```python
from build123d import *

# Parameters (mm, degrees)
SKETCH1_R                = 0.75
BOSS_EXTRUDE1_DEPTH      = 10
BOSS_EXTRUDE2_DEPTH      = 1.5
BOSS_EXTRUDE2_DEPTH_BACK = 1.5
FILLET1_R                = 1
SKETCH3_R                = 0.6
CUT_EXTRUDE1_DEPTH       = 5


with BuildPart() as part:
    # Sketch1 → Boss-Extrude1 (new body)
    with BuildSketch(Plane(origin=(0, 0, 0), x_dir=(0, 0, -1), z_dir=(1, 0, 0))):
        Circle(SKETCH1_R)
    extrude(amount=BOSS_EXTRUDE1_DEPTH)

    # Sketch2 → Boss-Extrude2 (add, two sides: drawn at the far end of the back side and taken through both)
    with BuildSketch(Plane(origin=(0, 0, 0), x_dir=(1, 0, 0), z_dir=(0, 1, 0)).offset(-BOSS_EXTRUDE2_DEPTH_BACK)):
        Polygon((1, 1.875), (1, -1.875), (-3, -1.875), (-3, -0.875), (0, -0.875), (0, 0.875), (-3, 0.875), (-3, 1.875), align=None)
    extrude(amount=BOSS_EXTRUDE2_DEPTH + BOSS_EXTRUDE2_DEPTH_BACK)

    # Fillet1
    fillet1_edges = [part.edges().sort_by_distance(p)[0] for p in [
        (-3, 1.5, 1.375),
        (-3, 1.5, -1.375),
        (-3, -1.5, -1.375),
        (1, 0, -1.875),
        (1, 0, 1.875),
        (-3, -1.5, 1.375),
    ]]
    fillet(fillet1_edges, radius=FILLET1_R)

    # Sketch3 → Cut-Extrude1 (cut)
    with BuildSketch(Plane(origin=(0, 0, -1.875), x_dir=(-1, 0, 0), z_dir=(0, 0, -1))):
        with Locations((1.7, 0)):
            Circle(SKETCH3_R)
    extrude(amount=-CUT_EXTRUDE1_DEPTH, mode=Mode.SUBTRACT)


solid = part.part
```
Work out the finished part from the listing and answer in its coordinate system (mm). A direction names the side the tool comes from. Round coordinates to 2 decimals unless told otherwise and drop trailing zeros. Write each loop counter-clockwise with the first axis right and the second up, starting at its lowest first coordinate (ties: lowest second). Pieces come first, ordered by that corner, then holes.
1) Determine the mould class of faces 1 (the face through (-0.9, 0, -1.875)), 2 (the face through (10, 0, 0)), 3 (the face through (0, 0, 0)) for opening direction Z: pulls with the +Z half, pulls with the -Z half, needs draft (parallel to the pull), parting line crosses it, or undercut.
2) A cutting plane is placed at B-B on x = -1.7. Determine the outline of the cut face in (y, z) (3 decimals), and give its area (3 significant figures).
3) A cutting plane is placed at A-A on y = 0. Determine the outline of the cut face in (x, z) (3 decimals), and give its area (3 significant figures).
4) Which of the six approach directions +Z, -Z, +X, -X, +Y, -Y give full straight-line access (tool end or side, diameter ignored) to faces 4 (the face through (-2.699, 1.215, -1.382)), 5 (the face through (1, -1, 0)), 6 (the face through (-0.8, 0, -0.875))?
5) Consider probe 1 along Y at (x, z) = (-1.7, -1.5); probe 2 along X at (y, z) = (-1, -0.25); probe 3 along Z at (x, y) = (-2, -0.85) (3 decimals). Determine where each line is inside the solid, lowest interval first.
6) A cutting plane is placed at C-C on z = 0. Determine the outline of the cut face in (x, y), and give its area (3 significant figures).
7) Flat-ended cylindrical pins translate along their axes: P1, Ø0.5, axis at y = 0.5, z = 0, coming from the -X side; P2, Ø2, axis at x = 4, z = 0, coming from the +Y side; P3, Ø1.5, axis at x = 6.5, z = 1, coming from the -Y side. Find the tip coordinate at first contact, or state that the pin passes through.
8) A cutting plane is placed at D-D on x = -0.25. Determine the outline of the cut face in (y, z) (3 decimals), and give its area (3 significant figures).
Entries:
1. face 1: pulls with the -Z half
1. face 2: needs draft
1. face 3: undercut
2. outline: (-1.5, -1.875) - (-0.6, -1.875) - (-0.6, -0.875) - (-1.5, -0.875) - close; (-1.5, 0.875) - (-0.6, 0.875) - (-0.6, 1.875) - (-1.5, 1.875) - close; (0.6, -1.875) - (1.5, -1.875) - (1.5, -0.875) - (0.6, -0.875) - close; (0.6, 0.875) - (1.5, 0.875) - (1.5, 1.875) - (0.6, 1.875) - close
2. area: 3.60 mm2
3. outline: (-3, -1.875) - (-2.3, -1.875) - (-2.3, -0.875) - (-3, -0.875) - close; (-3, 0.875) - (-2.3, 0.875) - (-2.3, 1.875) - (-3, 1.875) - close; (-1.1, -1.875) - (0, -1.875) arc R1 ccw to (1, -0.875) - (1, -0.75) - (10, -0.75) - (10, 0.75) - (1, 0.75) - (1, 0.875) arc R1 ccw to (0, 1.875) - (-1.1, 1.875) - (-1.1, 0.875) - (0, 0.875) - (0, -0.875) - (-1.1, -0.875) - close
3. area: 20.4 mm2
4. face 4: +Z, -Z, -X, +Y
4. face 5: +X
4. face 6: -X, +Y, -Y
5. probe 1: y = -1.5 to -0.6, 0.6 to 1.5
5. probe 2: x = 0 to 1
5. probe 3: z = -1.875 to -0.875, 0.875 to 1.875
6. outline: (0, -1.5) - (1, -1.5) - (1, -0.75) - (10, -0.75) - (10, 0.75) - (1, 0.75) - (1, 1.5) - (0, 1.5) - close
6. area: 16.5 mm2
7. P1: stops at x = 0
7. P2: stops at y = 0.75
7. P3: stops at y = -0.71
8. outline: (-1.5, -1.875) - (1.5, -1.875) - (1.5, -0.875) - (-1.5, -0.875) - close; (-1.5, 0.875) - (1.5, 0.875) - (1.5, 1.875) - (-1.5, 1.875) - close
8. area: 6.00 mm2
